The listing builds one solid part. Answer for the finished solid, in the listing's coordinates (mm). Face numbers are marked on the shaded views. A direction names the side the tool comes from. Give positions to 0.01 mm unless a question says otherwise; leave off trailing zeros. Write each loop counter-clockwise with the first axis right and the second up, starting at its lowest first coordinate (ties: lowest second). Pieces come first, ordered by that corner, then holes. Notation, with made-up numbers: (43, -25.75) - (99, -25.75) arc R26 cw to (99, -3.75) - close; hole circle Ø3 at (23, 75.25). An arc over 180 degrees is marked (long way). Write each question's results on one line, items separated by ' | '. Start each with the question number.
Q1. Section D-D (x = 98.5) is taken. Determine the outline of the cut face in (y, z) (3 decimals), plus the area to 3 significant figures.
Q2. Section A-A (z = 1.5) is taken. Determine the outline of the cut face in (x, y) (3 decimals).
Q3. Section B-B (x = 72) is taken. Determine the outline of the cut face in (y, z) (3 decimals).
Q4. Flat-ended cylindrical pins translate along their axes: pin 1 Ø8.5 at (y, z) = (-16, 18.5) entering from -X (3 decimals); pin 2 Ø10 at (x, z) = (-10, 42) entering from -Y; pin 3 Ø19 at (y, z) = (12.5, 15) entering from -X; pin 4 Ø3 at (x, y) = (54.5, -9) entering from -Z. Find the tip coordinate at first contact, or state that the pin passes through.
Q5. For the marked faces 1, 2, 3, 4 and 5, determine the directions among +Z, -Z, +X, -X, +Y, -Y from which every point of the face is accessible in a straight line to the end or side of a thin tool.
Q6. Find the intervals of material crossed by probe 1 along Y at (x, z) = (54.5, 52.5); probe 2 along Z at (x, y) = (98.5, 7) (3 decimals); probe 3 along Z at (x, y) = (-27, -20.5) (3 decimals), in increasing order.
Q7. For a pull along X with two mould halves and no side action, classify the marked faces 6, 7 and 8 as pulls with the +X half, pulls with the -X half, needs draft (parallel to the pull), parting line crosses it, or undercut.
Q8. Section C-C (y = 28.5) is taken. Determine the outline of the cut face in (x, z) (3 decimals), plus the area to 3 significant figures.
```python
from build123d import *

# Parameters (mm, degrees)
F1_DEPTH = 63.5
F0_W     = 25.4
F0_H     = 19.05
F2_DEPTH = 25.4
F3_DEPTH = 7.9375
F5_R     = 6.35


with BuildPart() as f1:
    # F0 (on Front) → F1 (new body, symmetric)
    with BuildSketch(Plane.XZ):
        Polygon((-41.275, 9.525), (-41.275, -9.525), (41.275, -9.525), (41.275, 9.525), (22.225, 9.525), align=None)
    extrude(amount=F1_DEPTH, both=True)

    # F0 (on Front) → F2 (join, symmetric)
    with BuildSketch(Plane.XZ):
        with BuildLine():
            Line((22.225, 9.525), (41.275, 9.525))
            Line((41.275, 9.525), (41.275, 27.8859981267))
            ThreePointArc((41.275, 27.8859981267), (44.2074063081, 37.078652451), (51.9212857985, 42.8752))
            Line((51.9212857985, 42.8752), (60.325, 42.8752))
            Line((60.325, 42.8752), (60.325, 61.9252))
            Line((60.325, 61.9252), (56.0216490022, 61.9252))
            add(Edge.make_bspline(
                [(56.0216490022, 61.9252), (55.893919841, 61.9013716142), (55.5783651285, 61.9228608195), (55.4305035678, 61.9252)],
                knots=[0.9415521493, 0.9415521493, 0.9415521493, 0.9415521493, 0.9942623024, 0.9942623024, 0.9942623024, 0.9942623024], degree=3))
            Line((55.4305035678, 61.9252), (55.3886373275, 61.9252))
            Line((55.3886373275, 61.9252), (49.3340956488, 61.9252))
            ThreePointArc((49.3340956488, 61.9252), (29.8303542806, 49.6435849131), (22.225, 27.8859981267))
            Line((22.225, 27.8859981267), (22.225, 9.525))
        make_face()
        with Locations((73.025, 52.4002)):
            Rectangle(F0_W, F0_H)
    extrude(amount=F2_DEPTH, both=True)

    # F0 (on Front) → F3 (join, symmetric)
    with BuildSketch(Plane.XZ):
        with BuildLine():
            add(Edge.make_bspline(
                [(-41.275, 9.525), (-41.4724777652, 33.4488657069), (28.8867726716, 58.916791613), (49.3340956488, 61.9252)],
                knots=[0, 0, 0, 0, 0.7515772095, 0.7515772095, 0.7515772095, 0.7515772095], degree=3))
            Line((-41.275, 9.525), (22.225, 9.525))
            Line((22.225, 9.525), (22.225, 27.8859981267))
            ThreePointArc((22.225, 27.8859981267), (29.8303542806, 49.6435849131), (49.3340956488, 61.9252))
        make_face()
    extrude(amount=F3_DEPTH, both=True)

    # F0 (on Front) → F4 (revolve)
    with BuildSketch(Plane.XZ):
        Polygon((85.725, 66.675), (85.725, 61.9252), (85.725, 42.8752), (85.725, 38.1), (111.125, 38.1), (111.125, 66.675), align=None)
    revolve(axis=Axis((85.725, 0, 50.0126), (0, 0, 1)))

    # F5
    f5_edges = [f1.edges().sort_by_distance(p)[0] for p in [
        (-41.275, -63.5, 0),
        (41.275, -63.5, 0),
        (41.275, 63.5, 0),
        (-41.275, 63.5, 0),
    ]]
    fillet(f5_edges, radius=F5_R)


solid = f1.part
```
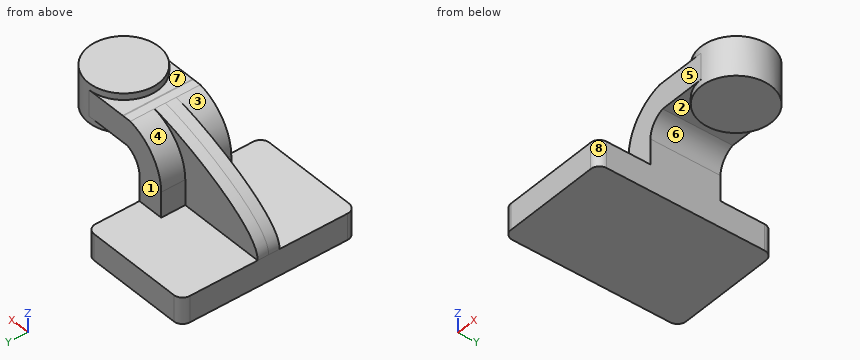
Answers below:
1) outline: (-21.954, 38.1) - (21.954, 38.1) - (21.954, 66.675) - (-21.954, 66.675) - close | area: 1,250 mm2
2) outline: (-41.275, -57.15) arc R6.35 ccw to (-34.925, -63.5) - (34.925, -63.5) arc R6.35 ccw to (41.275, -57.15) - (41.275, 57.15) arc R6.35 ccw to (34.925, 63.5) - (-34.925, 63.5) arc R6.35 ccw to (-41.275, 57.15) - close
3) outline: (-25.4, 42.875) - (-21.373, 42.875) - (-21.373, 38.1) - (21.373, 38.1) - (21.373, 42.875) - (25.4, 42.875) - (25.4, 61.925) - (21.373, 61.925) - (21.373, 66.675) - (-21.373, 66.675) - (-21.373, 61.925) - (-25.4, 61.925) - close
4) pin 1: stops at x = 22.225 | pin 2: stops at y = -7.94 | pin 3: stops at x = -41.28 | pin 4: stops at z = 42.88
5) face 1: +Z, +X, -X, +Y | face 2: -Z | face 3: +Z, -X, -Y | face 4: +Z, -X, +Y | face 5: +Z, +X, -X, -Y
6) probe 1: y = -25.4 to 25.4 | probe 2: z = 38.1 to 66.675 | probe 3: z = -9.525 to 9.525
7) face 6: undercut | face 7: needs draft | face 8: pulls with the +X half
8) outline: (-41.275, -9.525) - (41.275, -9.525) - (41.275, 9.525) - (-41.275, 9.525) - close | area: 1,570 mm2
